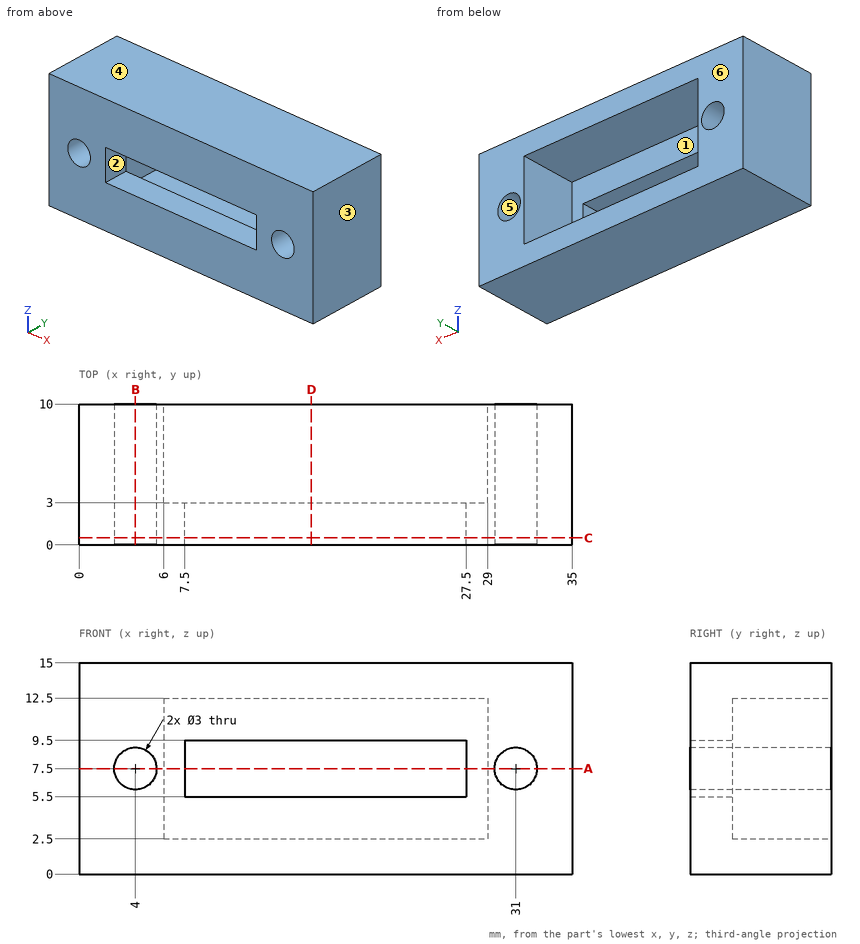
Verification items for this drawing (mm, ordinates from the low corner). A direction names the side the tool comes from. Coordinates: 2 decimals unless noted, no trailing zeros. Order: outer loops, then holes, each group sorted by start corner. A loop starts at its lowest first (then second) coordinate and runs counter-clockwise, first axis right, second up. Notation, with made-up numbers: (37, 76) - (78, 76) arc R24 cw to (78, 98) - close; hole circle Ø6 at (-13.5, 88). An arc over 180 degrees is marked (long way). Answer as a JSON object with one key per item and string values. Group by question number.
Item 1: Sectioned sample at A-A, the plane z = 7.5. Record the cut outline in (x, y), and give its area (3 significant figures).
Item 2: Sectioned sample at D-D, the plane x = 16.5. Record the cut outline in (y, z).
Item 3: Sectioned sample at B-B, the plane x = 4. Record the cut outline in (y, z), and give its area (3 significant figures).
Item 4: Draft check along Z on the marked faces 4, 5 and 6. Enter one of: +Z half, -Z half, draft (parallel to the pull), parting line (faces both ways), or undercut.
Item 5: Scan lines: probe 1 along X at (y, z) = (3.25, 7.5); probe 2 along Z at (x, y) = (17.5, 6.75); probe 3 along X at (y, z) = (9.25, 12). Record each from-to range of solid material in increasing order.
Item 6: Depth check by flat-ended pin: pin 1 Ø5 at (x, z) = (16.5, 6.5) entering from +Y. Enter the tip coordinate at first touch or a pass-through.
Item 7: Tool access check on the marked faces 1, 2 and 3. Record the directions out of +Z, -Z, +X, -X, +Y, -Y that give a thin tool (end or side, any length) a straight path to the whole face; none if there is none.
Item 8: Sectioned sample at C-C, the plane y = 0.5. Record the cut outline in (x, z).
Resolved:
{
 "1": {"outline": "(0, 0) - (2.5, 0) - (2.5, 10) - (0, 10) - close; (5.5, 0) - (7.5, 0) - (7.5, 3) - (6, 3) - (6, 10) - (5.5, 10) - close; (27.5, 0) - (29.5, 0) - (29.5, 10) - (29, 10) - (29, 3) - (27.5, 3) - close; (32.5, 0) - (35, 0) - (35, 10) - (32.5, 10) - close", "area": "69.0 mm^2"},
 "2": {"outline": "(0, 0) - (10, 0) - (10, 2.5) - (3, 2.5) - (3, 5.5) - (0, 5.5) - close; (0, 9.5) - (3, 9.5) - (3, 12.5) - (10, 12.5) - (10, 15) - (0, 15) - close"},
 "3": {"outline": "(0, 0) - (10, 0) - (10, 6) - (0, 6) - close; (0, 9) - (10, 9) - (10, 15) - (0, 15) - close", "area": "120 mm^2"},
 "4": {"face 4": "+Z half", "face 5": "undercut", "face 6": "draft"},
 "5": {"probe 1": "0 to 2.5, 5.5 to 6, 29 to 29.5, 32.5 to 35", "probe 2": "0 to 2.5, 12.5 to 15", "probe 3": "0 to 6, 29 to 35"},
 "6": {"pin 1": "y = 3"},
 "7": {"face 1": "+Y", "face 2": "+Y, -Y", "face 3": "+Z, -Z, +X, +Y, -Y"},
 "8": {"outline": "(0, 0) - (35, 0) - (35, 15) - (0, 15) - close; hole circle Ø3 at (4, 7.5); hole (7.5, 5.5) - (27.5, 5.5) - (27.5, 9.5) - (7.5, 9.5) - close; hole circle Ø3 at (31, 7.5)"}
}
